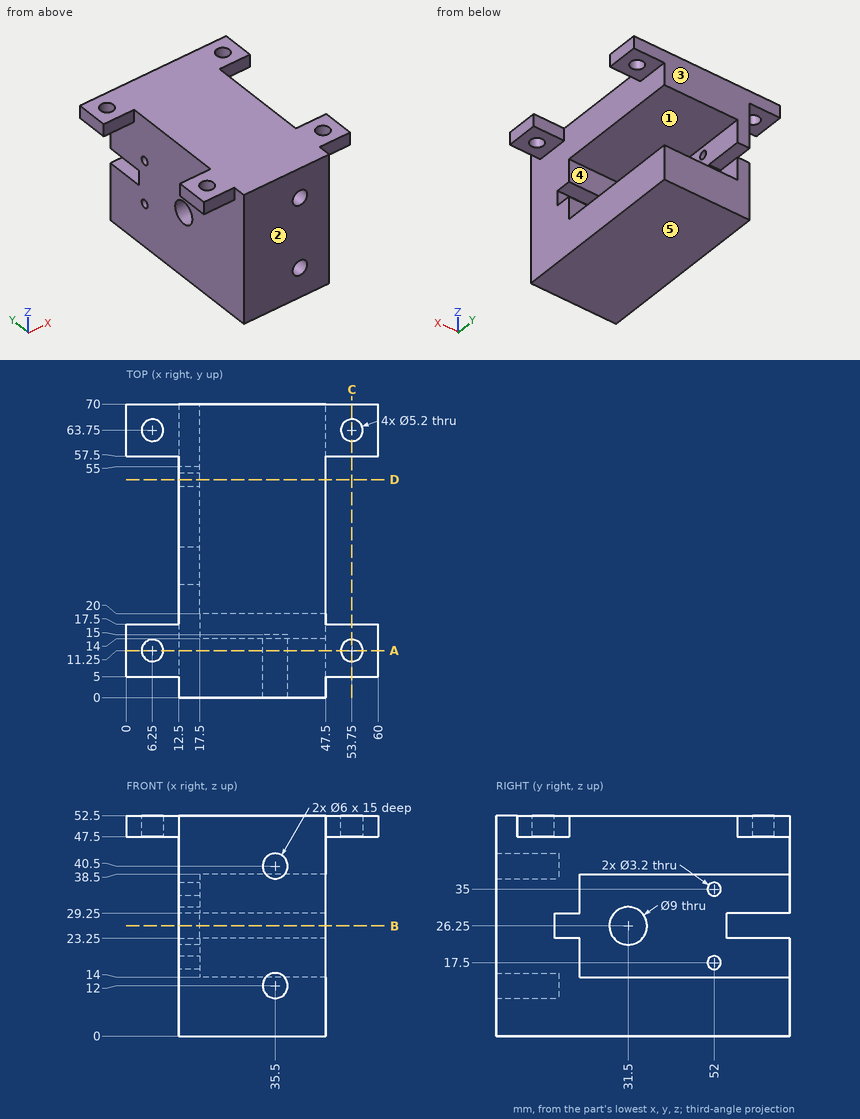
Geometry: see drawing. Coordinates: mm, zero at the bounding-box minimum. A direction names the side the tool comes from. Coordinates: 2 decimals unless noted, no trailing zeros. Order: outer loops, then holes, each group sorted by start corner. A loop starts at its lowest first (then second) coordinate and runs counter-clockwise, first axis right, second up. Notation, with made-up numbers: (6.5, -5.75) - (27.5, -5.75) arc R3 cw to (27.5, -0.75) - close; hole circle Ø10 at (53.25, 71). An arc over 180 degrees is marked (long way). Return JSON: item names as keys, results as strings.
Q1. First-contact query: pin 1 (10 mm diameter, centred on x = 55, y = 10, fed in from -Z); pin 2 (2 mm diameter, centred on y = 20, z = 19, fed in from -X); pin 3 (4 mm diameter, centred on y = 51.5, z = 28, fed in from +X). Flat tips, straight axial feed; report the tip coordinate or a pass-through.
The answers:
{"pin 1": "stops at z = 47.5", "pin 2": "stops at x = 12.5", "pin 3": "stops at x = 17.5"}
Q2. Draft query along Z for the marked faces 3, 4 and 5. Return one class per face: +Z half, -Z half, draft (parallel to the pull), parting line (faces both ways), or undercut.
The answers:
{"face 3": "draft", "face 4": "undercut", "face 5": "-Z half"}
Q3. Cut plane D-D (y = 52). Return loops of the section in (x, z), then the cut area to 3 significant figures.
The answers:
{"outline": "(12.5, 0) - (47.5, 0) - (47.5, 14) - (17.5, 14) - (17.5, 15.9) - (12.5, 15.9) - close; (12.5, 19.1) - (17.5, 19.1) - (17.5, 33.4) - (12.5, 33.4) - close; (12.5, 36.6) - (17.5, 36.6) - (17.5, 38.5) - (47.5, 38.5) - (47.5, 52.5) - (12.5, 52.5) - close", "area": "1,070 mm2"}
Q4. Access query for the marked faces 1 and 2. Directions: +Z, -Z, +X, -X, +Y, -Y. A direction counts if a zero-diameter tool reaches every point of the face in a straight line with its end or side. Return the directions, or none.
The answers:
{"face 1": "+X, +Y", "face 2": "+Z, -Z, +X, -X, -Y"}
Q5. Cut plane B-B (z = 26.25). Return loops of the section in (x, y), then the cut area to 3 significant figures.
The answers:
{"outline": "(12.5, 0) - (47.5, 0) - (47.5, 14) - (17.5, 14) - (17.5, 27) - (12.5, 27) - close; (12.5, 36) - (17.5, 36) - (17.5, 55) - (12.5, 55) - close", "area": "650 mm2"}
Q6. Ray query, probe 1 along Y at (x, z) = (6.25, 49.25); probe 2 along Z at (x, y) = (22.5, 66); probe 3 along Z at (x, y) = (16, 58.5). Return the intervals inside material, ascending.
The answers:
{"probe 1": "y = 5 to 8.65, 13.85 to 17.5, 57.5 to 61.15, 66.35 to 70", "probe 2": "z = 0 to 14, 38.5 to 52.5", "probe 3": "z = 0 to 23.25, 29.25 to 52.5"}
Q7. Cut plane A-A (y = 11.25). Return loops of the section in (x, z), then the cut area to 3 significant figures.
The answers:
{"outline": "(0, 47.5) - (3.65, 47.5) - (3.65, 52.5) - (0, 52.5) - close; (8.85, 47.5) - (12.5, 47.5) - (12.5, 0) - (47.5, 0) - (47.5, 47.5) - (51.15, 47.5) - (51.15, 52.5) - (8.85, 52.5) - close; (56.35, 47.5) - (60, 47.5) - (60, 52.5) - (56.35, 52.5) - close; hole circle Ø6 at (35.5, 12); hole circle Ø6 at (35.5, 40.5)", "area": "1,850 mm2"}
Q8. Cut plane C-C (x = 53.75). Return loops of the section in (y, z), then the cut area to 3 significant figures.
The answers:
{"outline": "(5, 47.5) - (8.65, 47.5) - (8.65, 52.5) - (5, 52.5) - close; (13.85, 47.5) - (17.5, 47.5) - (17.5, 52.5) - (13.85, 52.5) - close; (57.5, 47.5) - (61.15, 47.5) - (61.15, 52.5) - (57.5, 52.5) - close; (66.35, 47.5) - (70, 47.5) - (70, 52.5) - (66.35, 52.5) - close", "area": "73.0 mm2"}
